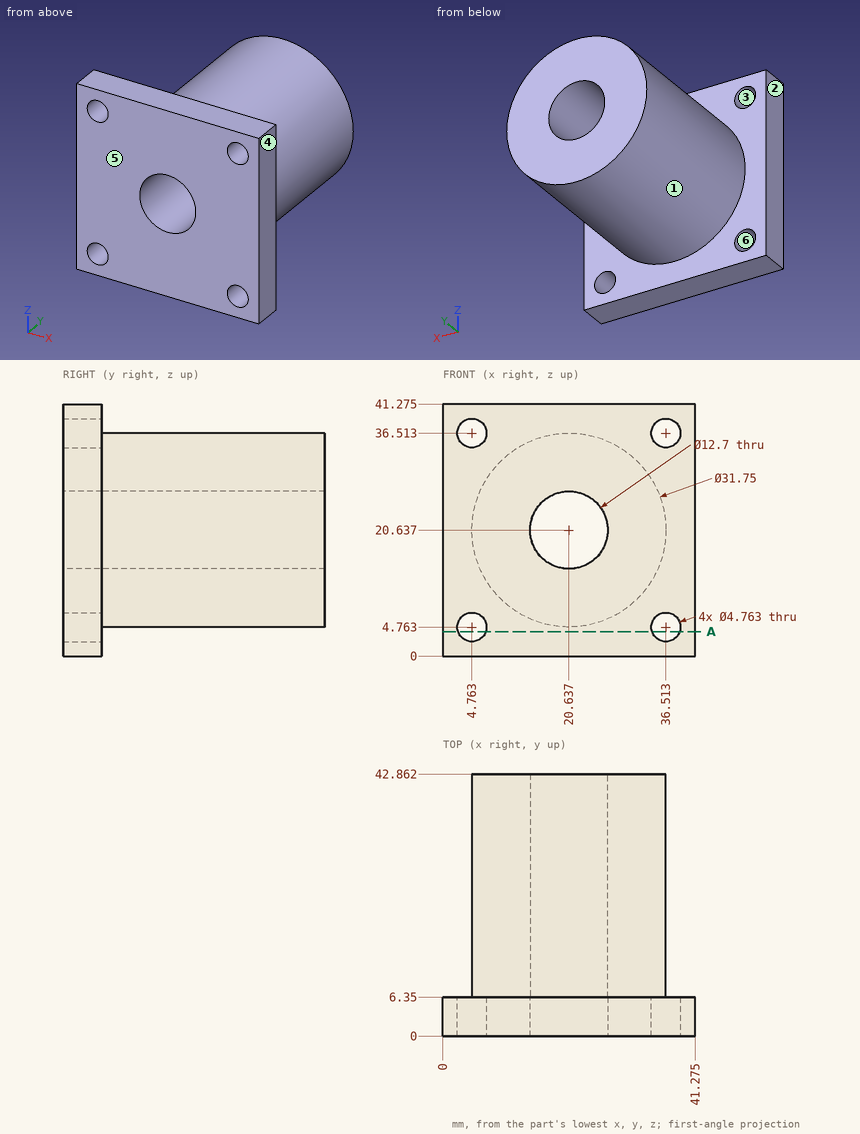
Answer from the drawing. Dimensions are ordinates in mm from the lowest x, y and z of the part. A direction names the side the tool comes from. Coordinates: 2 decimals unless noted, no trailing zeros. Answer as a JSON object with one key per item and string values.
1) Consider line 1 along Z through (x, y) = (38, 4) (1 decimal); line 2 along X through (y, z) = (3.5, 4) (1 decimal); line 3 along Z through (x, y) = (20.5, 9) (1 decimal). Determine where each line is inside the solid, lowest interval first. Write a range as from..to.
Model answer:
{"line 1": "z = 0..2.9, 6.6..34.7, 38.4..41.3", "line 2": "x = 0..2.5, 7..34.3, 38.8..41.3", "line 3": "z = 4.8..14.3, 27..36.5"}
2) Each of these flat-tipped pins is pushed along its axis until it touches: pin 1 (3 mm diameter, centred on y = 17.5, z = 9.5, fed in from -X); pin 2 (1 mm diameter, centred on x = 27, y = 8.5, fed in from +Z); pin 3 (4.5 mm diameter, centred on x = 4.76, z = 4.76, fed in from -Y); pin 4 (1 mm diameter, centred on x = 5.5, y = 16.5, fed in from +Z) (1 decimal). Where does it stop, or does it pass through?
Model answer:
{"pin 1": "stops at x = 8.02", "pin 2": "stops at z = 35.39", "pin 3": "passes through", "pin 4": "stops at z = 26.8"}
3) A tool of negligible diameter and unlimited length cuts with its end or side. For the marked faces 1 and 2, from which of +Z, -Z, +X, -X, +Y, -Y can it reach the whole face along a straight path? Write none if from no direction.
Model answer:
{"face 1": "+Y", "face 2": "+Z, -Z, -X, +Y, -Y"}
4) The mould has two halves that part along X. Classify the marked faces 3, 4, 5 and 6: released by +X, released by -X, zero draft, split by the parting line, or undercut.
Model answer:
{"face 3": "undercut", "face 4": "released by +X", "face 5": "zero draft", "face 6": "undercut"}
5) A cutting plane is placed at A-A, the plane z = 4. State how many separate pieces and enclosed holes the cut face has, plus the area to 3 significant figures.
Model answer:
{"separate pieces": "3", "enclosed holes": "0", "area": "205 mm²"}
